from build123d import *

# Parameters (mm, degrees)
BOSS_EXTRUDE1_DEPTH = 6.35
FILLET1_R           = 2


with BuildPart() as part:
    # Sketch1 → Boss-Extrude1 (new body)
    with BuildSketch(Plane(origin=(0, 0, 0), x_dir=(1, 0, 0), z_dir=(0, 1, 0))):
        Polygon((0, 0), (0, 10), (-6.7, 10), (-6.7, 16.35), (-26.7, 16.35), (-26.7, 10), (-51.7, 10), (-51.7, 16.35), (-71.7, 16.35), (-71.7, 10), (-96.7, 10), (-96.7, 16.35), (-116.7, 16.35), (-116.7, 10), (-141.7, 10), (-141.7, 16.35), (-161.7, 16.35), (-161.7, 10), (-166.7, 10), (-166.7, 0), (-166.7, -10), (-161.7, -10), (-161.7, -16.35), (-141.7, -16.35), (-141.7, -10), (-116.7, -10), (-116.7, -16.35), (-96.7, -16.35), (-96.7, -10), (-71.7, -10), (-71.7, -16.35), (-51.7, -16.35), (-51.7, -10), (-26.7, -10), (-26.7, -16.35), (-6.7, -16.35), (-6.7, -10), (0, -10), align=None)
    extrude(amount=BOSS_EXTRUDE1_DEPTH)

    # Fillet1
    fillet1_edges = [part.edges().sort_by_distance(p)[0] for p in [
        (-6.7, 3.175, 16.35),
        (-26.7, 3.175, 16.35),
        (-51.7, 3.175, 16.35),
        (-71.7, 3.175, 16.35),
        (-96.7, 3.175, 16.35),
        (-116.7, 3.175, 16.35),
        (-141.7, 3.175, 16.35),
        (-161.7, 3.175, 16.35),
        (-161.7, 3.175, -16.35),
        (-141.7, 3.175, -16.35),
        (-116.7, 3.175, -16.35),
        (-96.7, 3.175, -16.35),
        (-71.7, 3.175, -16.35),
        (-51.7, 3.175, -16.35),
        (-26.7, 3.175, -16.35),
        (-6.7, 3.175, -16.35),
    ]]
    fillet(fillet1_edges, radius=FILLET1_R)


solid = part.part
Check sheet for the modelled part. Datum: model origin and axes. Units: mm. A direction names the side the tool comes from. Round coordinates to 2 decimals unless told otherwise and drop trailing zeros. Loops run counter-clockwise (first coordinate to the right, second up) from the corner with the lowest first, then second, coordinate; pieces in that order, holes last. Notation, with made-up numbers: (65, -30.5) -> (108, -30.5) arc R21 cw to (108, -6.5) -> close; hole circle Ø4 at (-1, 17.5). An arc over 180 degrees is marked (long way). Put each result on its own line as item: value. Start each with the question number.
1. Access from +Z, -Z, +X, -X, +Y, -Y to the whole of each face (thin tool, end or side, straight path). Record for faces 1 (the face through (-51.7, 3, -12)), 2 (the face through (-141.7, 3, 12)), 3 (the face through (-6.7, 3, -12)).
2. Gauge pin test, flat ends, axial feed: pin 1 (2.5 mm diameter, centred on x = -163.5, y = 2.5, fed in from +Z); pin 2 (2.5 mm diameter, centred on x = -163.5, y = 4, fed in from -Z); pin 3 (2 mm diameter, centred on y = 4.5, z = 12, fed in from -X); pin 4 (5 mm diameter, centred on x = -66, z = 3.5, fed in from -Y). Record the tip position at first contact, or that the pin passes through.
3. Scan lines: probe 1 along X at (y, z) = (3, 12); probe 2 along Z at (x, y) = (-135, 5.5); probe 3 along X at (y, z) = (1.25, 15.5). Record each from-to range of solid material in increasing order.
4. Section check A-A (z = 12.5). Enter the section's corners in (x, y), plus the area to 3 significant figures.
5. Draft check along X on faces 4 (the face through (-6.7, 3, 12)), 5 (the face through (-84, 3, 10)), 6 (the face through (-62, 3, -16.35)). Enter one of: +X half, -X half, draft (parallel to the pull), parting line (faces both ways), or undercut.
6. Section check B-B (x = -46). Enter the section's corners in (y, z).
Findings:
1. face 1: -Z, +Y, -Y
1. face 2: +Z, +Y, -Y
1. face 3: -Z, +X, +Y, -Y
2. pin 1: stops at z = 10
2. pin 2: stops at z = -10
2. pin 3: stops at x = -161.7
2. pin 4: stops at y = 0
3. probe 1: x = -161.7 to -141.7, -116.7 to -96.7, -71.7 to -51.7, -26.7 to -6.7
3. probe 2: z = -10 to 10
3. probe 3: x = -161.34 to -142.06, -116.34 to -97.06, -71.34 to -52.06, -26.34 to -7.06
4. outline: (-161.7, 0) -> (-141.7, 0) -> (-141.7, 6.35) -> (-161.7, 6.35) -> close; (-116.7, 0) -> (-96.7, 0) -> (-96.7, 6.35) -> (-116.7, 6.35) -> close; (-71.7, 0) -> (-51.7, 0) -> (-51.7, 6.35) -> (-71.7, 6.35) -> close; (-26.7, 0) -> (-6.7, 0) -> (-6.7, 6.35) -> (-26.7, 6.35) -> close
4. area: 508 mm^2
5. face 4: +X half
5. face 5: undercut
5. face 6: draft
6. outline: (0, -10) -> (6.35, -10) -> (6.35, 10) -> (0, 10) -> close
